Design review of the part shown in the three views and the two pictorial views. Dimensions are in mm from the part's minimum x, y and z. A direction names the side the tool comes from. Give positions to 0.01 mm unless a question says otherwise; leave off trailing zeros. Loops run counter-clockwise (first coordinate to the right, second up) from the corner with the lowest first, then second, coordinate; pieces in that order, holes last. Notation, with made-up numbers: (75.5, -39.5) - (93.5, -39.5) arc R33 cw to (93.5, -1.5) - close; hole circle Ø4 at (71, 60). An arc over 180 degrees is marked (long way). Answer as a JSON object with one key per item and string values.
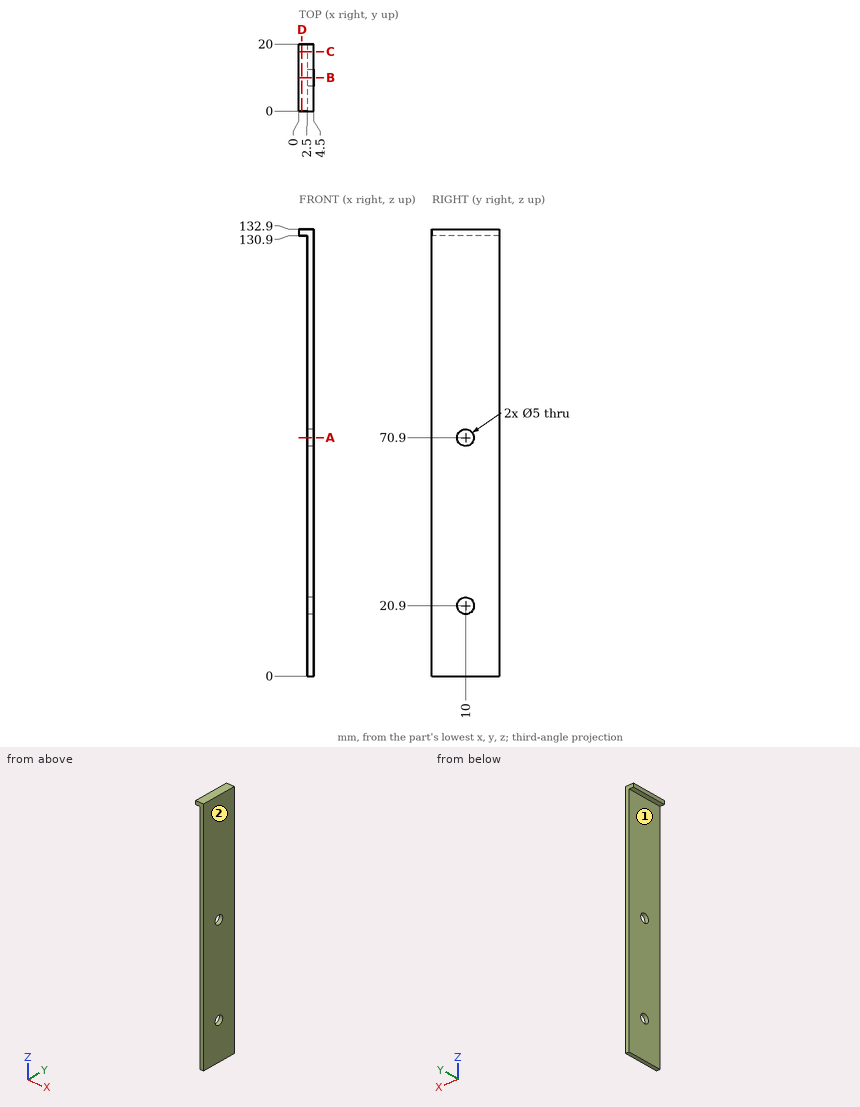
Q1. Clearance check with a flat-ended pin moving along its axis: pin 1 Ø6 at (y, z) = (9.5, 99.5) entering from -X. State where the tip first meets the part, or that it passes through.
Results:
{"pin 1": "stops at x = 2.5"}
Q2. Consider section B-B, the plane y = 10. State the section outline as (x, z) points.
Results:
{"outline": "(0, 130.9) - (2.5, 130.9) - (2.5, 73.4) - (4.5, 73.4) - (4.5, 132.9) - (0, 132.9) - close; (2.5, 0) - (4.5, 0) - (4.5, 18.4) - (2.5, 18.4) - close; (2.5, 23.4) - (4.5, 23.4) - (4.5, 68.4) - (2.5, 68.4) - close"}
Q3. To check wall thickness, follow probe 1 along Z at (x, y) = (3.35, 10); probe 2 along Y at (x, z) = (3.15, 20.9); probe 3 along Z at (x, y) = (2.55, 9). State the ranges of each line that lie inside material, in increasing order. Write a range as [from, to].
Results:
{"probe 1": "z = [0, 18.4], [23.4, 68.4], [73.4, 132.9]", "probe 2": "y = [0, 7.5], [12.5, 20]", "probe 3": "z = [0, 18.61], [23.19, 68.61], [73.19, 132.9]"}
Q4. For the marked faces 1 and 2, list the 3-axis set-ups (+Z, -Z, +X, -X, +Y, -Y) from which the entire face can be reached by the end or side of a thin tool; tool diameter is ignored.
Results:
{"face 1": "-Z, -X, +Y, -Y", "face 2": "+Z, -Z, +X, +Y, -Y"}
Q5. Consider section D-D, the plane x = 0.9. State the section outline as (y, z) points.
Results:
{"outline": "(0, 130.9) - (20, 130.9) - (20, 132.9) - (0, 132.9) - close"}
Q6. Consider section A-A, the plane z = 70.9. State the section outline as (x, y) points, plus the area to 3 significant figures.
Results:
{"outline": "(2.5, 0) - (4.5, 0) - (4.5, 7.5) - (2.5, 7.5) - close; (2.5, 12.5) - (4.5, 12.5) - (4.5, 20) - (2.5, 20) - close", "area": "30.0 mm^2"}
Q7. Consider section C-C, the plane y = 17.75. State the section outline as (x, z) points.
Results:
{"outline": "(0, 130.9) - (2.5, 130.9) - (2.5, 0) - (4.5, 0) - (4.5, 132.9) - (0, 132.9) - close"}
